For this review, take the finished solid that the model builds, in its own axes (mm). A direction names the side the tool comes from. Coordinates: 2 decimals unless noted, no trailing zeros. Write each loop counter-clockwise with the first axis right and the second up, starting at its lowest first coordinate (ties: lowest second). Pieces come first, ordered by that corner, then holes.
1) For faces 4 (the face through (-4.72, -8.25, -3.01)), 5 (the face through (0, 5, 17)), 6 (the face through (0, 2, -63)), list the 3-axis set-ups (+Z, -Z, +X, -X, +Y, -Y) from which the entire face can be reached by the end or side of a thin tool; tool diameter is ignored.
2) We need section C-C on y = 4.25. Write out the cut boundary in (x, z).
3) We need section A-A on x = 0. Give the number of separate pieces and of enclosed holes in the cut face, then the cut area to 3 significant figures.
4) We need section B-B on z = 0. Write out the cut boundary in (x, y), then the cut area to 3 significant figures.
5) Mouldability with a two-part tool opening along X and no side actions: class faces 1 (the face through (2.6, -5.33, -1.35)), 2 (the face through (-7.94, 0, -18)), 3 (the face through (0, 1.5, 21)) as pulls with the +X half, pulls with the -X half, needs draft (parallel to the pull), parting line crosses it, or undercut.
6) To check wall thickness, follow line 1 along Z through (x, y) = (0, 5); line 2 along X through (y, z) = (-8.2, 0); line 3 along Z through (x, y) = (0, -2.5). State the ranges of each line that lie inside material, in increasing order.
7) We need section D-D on x = -7. Write out the cut boundary in (y, z).
8) Insertion check: P1, Ø5, axis at x = 0, z = -45.07, coming from the +Y side; P2, Ø6.5, axis at x = -2.5, z = 22, coming from the +Y side; P3, Ø5.5, axis at x = 0.5, y = 6, coming from the +Z side. Each pin has a flat end and moves straight along its axis. Give the tip position at first contact, or say it passes through.
from build123d import *

# Parameters (mm, degrees)
RESSALTO_EXTRUS_O1_DEPTH             = 7.94
FILETE1_R                            = 5
ESCAREADO_PARA_SFHCS_M51_AT_2_COUNT  = 2
ESCAREADO_PARA_SFHCS_M51_AT_2_PITCH  = 45.072604626
ESCAREADO_PARA_SFHCS_M51_AT_3_COUNT  = 2
ESCAREADO_PARA_SFHCS_M51_AT_3_PITCH  = 80.029473244
ESCAREADO_PARA_SFHCS_M51_AT_4_COUNT  = 2
ESCAREADO_PARA_SFHCS_M51_AT_4_PITCH  = 73.938988881
ESCAREADO_PARA_SFHCS_M52_D           = 5.5
ESCAREADO_PARA_SFHCS_M52_CSINK_D     = 11.2
ESCAREADO_PARA_SFHCS_M52_CSINK_ANGLE = 90


with BuildPart() as part:
    # Esboço1 → Ressalto-extrusão1 (new, symmetric)
    with BuildSketch(Plane(origin=(0, 0, 0), x_dir=(0, 0, -1), z_dir=(1, 0, 0))):
        Polygon((-17, -8.5), (63, -8.5), (63, 8.5), (-17, 8.5), (-17, 1.5), (-25, 1.5), (-25, -8.5), align=None)
    extrude(amount=RESSALTO_EXTRUS_O1_DEPTH, both=True)

    # Filete1
    filete1_edges = [part.edges().sort_by_distance(p)[0] for p in [
        (0, -8.5, -63),
        (0, -8.5, 25),
    ]]
    fillet(filete1_edges, radius=FILETE1_R)

    # Esboço3 → Escareado para SFHCS M51 (revolve, cut)
    with BuildSketch(Plane(origin=(0, -8.5, -45.072604626), x_dir=(0, 0, -1), z_dir=(1, 0, 0))):
        Polygon((0, 0), (0, 31.652366702), (2.75, 30), (2.75, 3.35), (5.6, 0.5), (5.6, 0), align=None)
    escareado_para_sfhcs_m51 = revolve(axis=Axis((0, -14.85, -45.072604626), (0, 1, 0)), mode=Mode.SUBTRACT)

    # Escareado para SFHCS M51 at 2: Escareado para SFHCS M51 ×2
    with Locations(*[(0, 0, i * ESCAREADO_PARA_SFHCS_M51_AT_2_PITCH) for i in range(1, ESCAREADO_PARA_SFHCS_M51_AT_2_COUNT)]):
        add(escareado_para_sfhcs_m51, mode=Mode.SUBTRACT)

    # Escareado para SFHCS M51 at 3: Escareado para SFHCS M51 ×2
    with Locations(*[Vector(-0.8263205706487303, 0, 0.563200066160114) * (i * ESCAREADO_PARA_SFHCS_M51_AT_3_PITCH) for i in range(1, ESCAREADO_PARA_SFHCS_M51_AT_3_COUNT)]):
        add(escareado_para_sfhcs_m51, mode=Mode.SUBTRACT)

    # Escareado para SFHCS M51 at 4: Escareado para SFHCS M51 ×2
    with Locations(*[Vector(-0.894386047210078, 0, 0.44729587361827106) * (i * ESCAREADO_PARA_SFHCS_M51_AT_4_PITCH) for i in range(1, ESCAREADO_PARA_SFHCS_M51_AT_4_COUNT)]):
        add(escareado_para_sfhcs_m51, mode=Mode.SUBTRACT)

    # Escareado para SFHCS M52 (through all)
    with Locations(Plane(origin=(0, -8.5, 0), x_dir=(-1, 0, 0), z_dir=(0, -1, 0))):
        with Locations((0, 22.887127338)):
            CounterSinkHole(ESCAREADO_PARA_SFHCS_M52_D / 2, ESCAREADO_PARA_SFHCS_M52_CSINK_D / 2, counter_sink_angle=ESCAREADO_PARA_SFHCS_M52_CSINK_ANGLE)


solid = part.part
Result:
1. face 4: -Y
1. face 5: +Z, +X, -X, +Y
1. face 6: -Z, +X, -X, +Y, -Y
2. outline: (-7.94, -63) - (7.94, -63) - (7.94, 17) - (-7.94, 17) - close; hole circle Ø5.5 at (0, -45.07); hole circle Ø5.5 at (0, -22.89); hole circle Ø5.5 at (0, 0)
3. separate pieces: 4
3. enclosed holes: 0
3. area: 1,120 mm2
4. outline: (-7.94, -8.5) - (-5.6, -8.5) - (-5.6, -8) - (-2.75, -5.15) - (-2.75, 8.5) - (-7.94, 8.5) - close; (2.75, -5.15) - (5.6, -8) - (5.6, -8.5) - (7.94, -8.5) - (7.94, 8.5) - (2.75, 8.5) - close
4. area: 165 mm2
5. face 1: undercut
5. face 2: pulls with the -X half
5. face 3: needs draft
6. line 1: z = -63 to -47.82, -42.32 to -25.64, -20.14 to -2.75, 2.75 to 17
6. line 2: x = -7.94 to -5.6, 5.6 to 7.94
6. line 3: z = -63 to -47.82, -42.32 to -25.64, -20.14 to -2.75, 2.75 to 25
7. outline: (-8.5, -58) arc R5 ccw to (-3.5, -63) - (8.5, -63) - (8.5, 17) - (1.5, 17) - (1.5, 25) - (-3.5, 25) arc R5 ccw to (-8.5, 20) - close
8. P1: passes through
8. P2: stops at y = 1.5
8. P3: stops at z = 17
